Solid Edge part; units mm, degrees
sketch "Sketch1" plane through (0, 0, 0) normal (0, -1, 0) x (1, 0, 0)
  circle A0 centre (0, 0) radius 100
extrude "Protrusion1" add sketch "Sketch1" against normal blind 150
sketch "Sketch2" plane through (0, 150, 0) normal (0, 1, 0) x (0, 0, 1)
  circle A0 centre (0, 0) radius 95
extrude "Recorte_Extrudado_2" cut sketch "Sketch2" against normal blind 251.4861
extrude "Recorte_Extrudado_3" [suppressed]
chamfer "Chanfro_1" distance 2 angle 45 1 edges at (0, 150, -95)
fillet "Redondo_1" [suppressed]
extrude "Recorte_Extrudado_5" [suppressed]
sketch "Sketch3" plane through (0, 0, 0) normal (0, -1, 0) x (1, 0, 0)
  circle A0 centre (0, 0) radius 100
extrude "Protrusão_Extrudada_5" add sketch "Sketch3" against normal blind 3
sketch "Sketch4" plane through (0, 0, 0) normal (0, 0, -1) x (-1, 0, 0)
  line L0 (-30, 40) -> (30, 40)
  line L1 (30, 40) -> (30, 260)
  line L2 (30, 260) -> (-30, 260)
  line L3 (-30, 260) -> (-30, 40)
extrude "Recorte_Extrudado_6" cut sketch "Sketch4" along normal mid plane 236.9884
sketch "Sketch5" plane through (0, 0, 0) normal (1, 0, 0) x (0, 1, 0)
  line L0 (65, 0) -> (65, 15)
  line L1 (65, 15) -> (33, 15)
  line L2 (33, 15) -> (33, -15)
  line L3 (33, -15) -> (65, -15)
  line L4 (65, -15) -> (65, 0)
extrude "Recorte_Extrudado_7" cut sketch "Sketch5" along normal blind 114.5948 and the other way blind 44.7082
sketch "Sketch6" plane through (0, 0, 0) normal (1, 0, 0) x (0, 1, 0)
  line L0 (150, 75.3939) -> (40, 75.3939)
  line L1 (40, 75.3939) -> (40, 50.3939)
  line L2 (40, 50.3939) -> (150, 50.3939)
  line L3 (150, 50.3939) -> (150, 75.3939)
  line L4 (150, -75.3939) -> (40, -75.3939)
  line L5 (40, -75.3939) -> (40, -50.3939)
  line L6 (40, -50.3939) -> (150, -50.3939)
  line L7 (150, -50.3939) -> (150, -75.3939)
extrude "Recorte_Extrudado_8" cut sketch "Sketch6" along normal mid plane 298.4716
sketch "Sketch7" plane through (-91.4411, 150, 0) normal (0, 1, 0) x (1, 0, 0)
  circle A0 centre (91.4411, 0) radius 100
extrude "Protrusão_Extrudada_6" add sketch "Sketch7" against normal blind 5
sketch "Sketch8" plane through (0, 150, 0) normal (0, 1, 0) x (0, 0, -1)
  circle A0 centre (0, 0) radius 90
extrude "Recorte_Extrudado_10" cut sketch "Sketch8" against normal up to vertex (5 mm away) and the other way blind 10.5295
Geometry: final body of the model. Coordinates: model frame, mm. A direction names the side the tool comes from. Round coordinates to 2 decimals unless told otherwise and drop trailing zeros. Loops run counter-clockwise (first coordinate to the right, second up) from the corner with the lowest first, then second, coordinate; pieces in that order, holes last. Notation, with made-up numbers: (50.25, 59.25) -> (83.25, 59.25) arc R16 cw to (83.25, 77.25) -> close; hole circle Ø1 at (-6.5, 31). An arc over 180 degrees is marked (long way). One line per question, with ' | ' between items. Start each with the question number.
1. Section B-B on y = 74. Output: boundary loops of the cut face in (x, z), and give its area (3 significant figures).
2. Line query: line 1 along X through (y, z) = (147, 0); line 2 along Y through (x, z) = (-41, -81); line 3 along X through (y, z) = (115.5, 0). Output: solid intervals per line, ascending. Write a range as [from, to].
3. Section D-D on x = -74.5. Output: boundary loops of the cut face in (y, z), and give its area (3 significant figures).
4. Set-up query: faces 1 (the face through (-13.6, 145, -89.4)), 2 (the face through (96, 49, 15)), 3 (the face through (-73, 40, 63)). Return all of +Z, -Z, +X, -X, +Y, -Y with unobstructed straight access to the full face (end or side cutting, diameter ignored); none if empty.
5. Contact query for flat-ended pins moving along their axis: pin 1 (4 mm diameter, centred on x = 61, y = 111, fed in from -Z); pin 2 (4.5 mm diameter, centred on x = 84.5, y = 116.5, fed in from -Z); pin 3 (5 mm diameter, centred on x = 61.5, z = -30, fed in from +Y); pin 4 (3 mm diameter, centred on x = -4.5, z = 43, fed in from -Y). Output: stop coordinate, or through.
6. Section C-C on x = 0. Output: boundary loops of the cut face in (y, z).
7. Mould query, pull axis Z, two halves, no side actions, for faces 4 (the face through (-73, 40, -63)), 5 (the face through (83, 92, -50.394)), 6 (the face through (62, 93, -75.394)), 7 (the face through (-30, 92, -93)). Classes: pulls with the +Z half, pulls with the -Z half, needs draft (parallel to the pull), parting line crosses it, or undercut.
8. Section A-A on z = 0. Output: boundary loops of the cut face in (x, y), and give its area (3 significant figures).
Returned:
1) outline: (-86.37, -50.39) -> (-80.53, -50.39) arc R95 cw to (-80.53, 50.39) -> (-86.37, 50.39) arc R100 ccw to start; (-65.69, -75.39) arc R100 ccw to (-30, -95.39) -> (-30, -90.14) arc R95 cw to (-57.8, -75.39) -> close; (-65.69, 75.39) -> (-57.8, 75.39) arc R95 cw to (-30, 90.14) -> (-30, 95.39) arc R100 ccw to start; (30, -95.39) arc R100 ccw to (65.69, -75.39) -> (57.8, -75.39) arc R95 cw to (30, -90.14) -> close; (30, 90.14) arc R95 cw to (57.8, 75.39) -> (65.69, 75.39) arc R100 ccw to (30, 95.39) -> close; (80.53, -50.39) -> (86.37, -50.39) arc R100 ccw to (86.37, 50.39) -> (80.53, 50.39) arc R95 cw to start | area: 1,790 mm2
2) line 1: x = [-100, -90], [90, 100] | line 2: y = [0, 3], [145, 150] | line 3: x = [-100, -95], [95, 100]
3) outline: (0, -66.71) -> (40, -66.71) -> (40, -58.95) -> (3, -58.95) -> (3, 58.95) -> (40, 58.95) -> (40, 66.71) -> (0, 66.71) -> close; (145, -66.71) -> (150, -66.71) -> (150, -50.5) -> (145, -50.5) -> close; (145, 50.5) -> (150, 50.5) -> (150, 66.71) -> (145, 66.71) -> close | area: 1,140 mm2
4) face 1: none | face 2: +X | face 3: +X, -X
5) pin 1: stops at z = -80.74 | pin 2: stops at z = -50.39 | pin 3: stops at y = 3 | pin 4: stops at y = 0
6) outline: (0, -100) -> (40, -100) -> (40, -95) -> (3, -95) -> (3, 95) -> (40, 95) -> (40, 100) -> (0, 100) -> close; (145, -100) -> (150, -100) -> (150, -90) -> (145, -90) -> close; (145, 90) -> (150, 90) -> (150, 100) -> (145, 100) -> close
7) face 4: undercut | face 5: pulls with the -Z half | face 6: undercut | face 7: needs draft
8) outline: (-100, 0) -> (100, 0) -> (100, 33) -> (95, 33) -> (95, 3) -> (-95, 3) -> (-95, 145) -> (-90, 145) -> (-90, 150) -> (-100, 150) -> close; (90, 145) -> (95, 145) -> (95, 65) -> (100, 65) -> (100, 150) -> (90, 150) -> close | area: 1,960 mm2
